Check sheet for the drawn part. Datum: minimum x, y, z corner. Units: mm. A direction names the side the tool comes from. Coordinates: 2 decimals unless noted, no trailing zeros. Loops run counter-clockwise (first coordinate to the right, second up) from the corner with the lowest first, then second, coordinate; pieces in that order, holes last. Notation, with made-up numbers: (57.25, 87.25) - (79.25, 87.25) arc R32 cw to (79.25, 118.25) - close; hole circle Ø9 at (74, 22). An arc over 180 degrees is marked (long way). Write item = value, one per line. Start each with the question number.
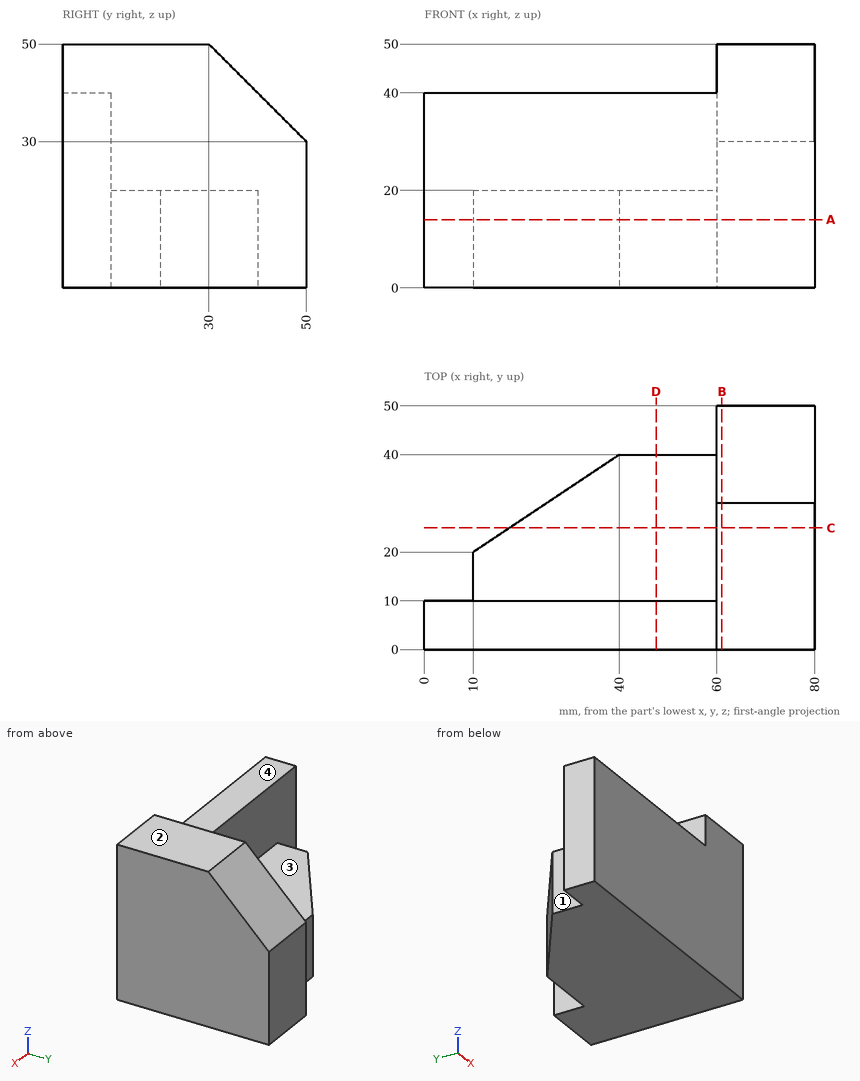
(1) Scan lines: line 1 (Z direction, x = 53, y = 4); line 2 (X direction, y = 19.5, z = 3); line 3 (Z direction, x = 29, y = 14). Record each from-to range of solid material in increasing order.
(2) Sectioned sample at B-B on x = 61. Enter the section's corners in (y, z).
(3) Sectioned sample at D-D on x = 47.5. Enter the section's corners in (y, z).
(4) Tool access check on the marked faces 1, 2, 3 and 4. Record the directions out of +Z, -Z, +X, -X, +Y, -Y that give a thin tool (end or side, any length) a straight path to the whole face; none if there is none.
(5) Sectioned sample at A-A on z = 14. Enter the section's corners in (x, y).
(6) Depth check by flat-ended pin: pin 1 (6 mm diameter, centred on x = 12, y = 7, fed in from +Z); pin 2 (11 mm diameter, centred on y = 16.5, z = 11, fed in from -X); pin 3 (3 mm diameter, centred on x = 56, y = 42, fed in from +Z); pin 4 (15 mm diameter, centred on x = 25, y = 31, fed in from +Z). Enter the tip coordinate at first touch or a pass-through.
(7) Sectioned sample at C-C on y = 25. Enter the section's corners in (x, z).
Working result:
q1.line_1 = 0 to 40
q1.line_2 = 10 to 80
q1.line_3 = 0 to 20
q2.outline = (0, 0) - (50, 0) - (50, 30) - (30, 50) - (0, 50) - close
q3.outline = (0, 0) - (40, 0) - (40, 20) - (10, 20) - (10, 40) - (0, 40) - close
q4.face_1 = +Z, -Z, -X, +Y
q4.face_2 = +Z, +X, -X, +Y, -Y
q4.face_3 = +Z, -X, +Y
q4.face_4 = +Z, -X, +Y, -Y
q5.outline = (0, 0) - (80, 0) - (80, 50) - (60, 50) - (60, 40) - (40, 40) - (10, 20) - (10, 10) - (0, 10) - close
q6.pin_1 = 40
q6.pin_2 = 10
q6.pin_3 = through
q6.pin_4 = 20
q7.outline = (17.5, 0) - (80, 0) - (80, 50) - (60, 50) - (60, 20) - (17.5, 20) - close
